from build123d import *

# Parameters (mm, degrees)
F1_DEPTH = 2


with BuildPart() as f1:
    # F0 (on Front) → F1 (new body)
    with BuildSketch(Plane.XZ):
        with BuildLine():
            Line((-13.003751, 47.985914), (-13.003751, 17.985914))
            Line((-13.003751, 17.985914), (-13.003751, -0.014086))
            Line((-13.003751, -0.014086), (-15.003751, -0.014086))
            Line((-15.003751, -0.014086), (-15.003751, 8.985914))
            Line((-15.003751, 8.985914), (-17.003751, 8.985914))
            ThreePointArc((-17.003751, 8.985914), (-18.417965, 8.400127), (-19.003751, 6.985914))
            Line((-19.003751, 6.985914), (-19.003751, -6.014086))
            Line((-19.003751, -6.014086), (-20.003751, -6.014086))
            Line((-20.003751, -6.014086), (-20.003751, -8.764086))
            Line((-20.003751, -8.764086), (-25.003751, -8.764086))
            ThreePointArc((-25.003751, -8.764086), (-26.417965, -9.349873), (-27.003751, -10.764086))
            Line((-27.003751, -10.764086), (-27.003751, -13.014086))
            Line((-27.003751, -13.014086), (-21.003751, -13.014086))
            Line((-21.003751, -13.014086), (-21.003751, -15.014086))
            Line((-21.003751, -15.014086), (-27.003751, -15.014086))
            Line((-27.003751, -15.014086), (-27.003751, -17.264086))
            ThreePointArc((-27.003751, -17.264086), (-26.417965, -18.6783), (-25.003751, -19.264086))
            Line((-25.003751, -19.264086), (-18.877196, -19.264086))
            Line((-18.877196, -19.264086), (-18.877196, -22.014086))
            Line((-18.877196, -22.014086), (-15.003751, -22.014086))
            ThreePointArc((-15.003751, -22.014086), (-13.589538, -21.4283), (-13.003751, -20.014086))
            Line((-13.003751, -20.014086), (-13.003751, -16.266214))
            ThreePointArc((-13.003751, -16.266214), (-12.094926, -14.590106), (-10.194413, -14.437287))
            ThreePointArc((-10.194413, -14.437287), (1.996249, -17.014086), (14.18691, -14.437287))
            ThreePointArc((14.18691, -14.437287), (16.087423, -14.590106), (16.996249, -16.266214))
            Line((16.996249, -16.266214), (16.996249, -20.014086))
            ThreePointArc((16.996249, -20.014086), (17.582035, -21.4283), (18.996249, -22.014086))
            Line((18.996249, -22.014086), (22.869694, -22.014086))
            Line((22.869694, -22.014086), (22.869694, -19.264086))
            Line((22.869694, -19.264086), (28.996249, -19.264086))
            ThreePointArc((28.996249, -19.264086), (30.410462, -18.6783), (30.996249, -17.264086))
            Line((30.996249, -17.264086), (30.996249, -15.014086))
            Line((30.996249, -15.014086), (24.996249, -15.014086))
            Line((24.996249, -15.014086), (24.996249, -13.014086))
            Line((24.996249, -13.014086), (30.996249, -13.014086))
            Line((30.996249, -13.014086), (30.996249, -10.764086))
            ThreePointArc((30.996249, -10.764086), (30.410462, -9.349873), (28.996249, -8.764086))
            Line((28.996249, -8.764086), (23.996249, -8.764086))
            Line((23.996249, -8.764086), (23.996249, -6.014086))
            Line((23.996249, -6.014086), (22.996249, -6.014086))
            Line((22.996249, -6.014086), (22.996249, 6.985914))
            ThreePointArc((22.996249, 6.985914), (22.410462, 8.400127), (20.996249, 8.985914))
            Line((20.996249, 8.985914), (18.996249, 8.985914))
            Line((18.996249, 8.985914), (18.996249, -0.014086))
            Line((18.996249, -0.014086), (16.996249, -0.014086))
            Line((16.996249, -0.014086), (16.996249, 17.985914))
            Line((16.996249, 17.985914), (16.996249, 47.985914))
            ThreePointArc((16.996249, 47.985914), (16.410462, 49.400127), (14.996249, 49.985914))
            Line((14.996249, 49.985914), (-11.003751, 49.985914))
            ThreePointArc((-11.003751, 49.985914), (-12.417965, 49.400127), (-13.003751, 47.985914))
        make_face()
        with BuildLine():
            Line((2.996249, -12.014086), (0.996249, -12.014086))
            Line((0.996249, -12.014086), (0.996249, -9.014086))
            ThreePointArc((0.996249, -9.014086), (1.996249, -0.126604), (2.996249, -9.014086))
            Line((2.996249, -9.014086), (2.996249, -12.014086))
        make_face(mode=Mode.SUBTRACT)
        with BuildLine():
            ThreePointArc((-8.503751, 37.985914), (-7.917965, 39.400127), (-6.503751, 39.985914))
            Line((-6.503751, 39.985914), (10.496249, 39.985914))
            ThreePointArc((10.496249, 39.985914), (11.910462, 39.400127), (12.496249, 37.985914))
            Line((12.496249, 37.985914), (12.496249, 19.985914))
            ThreePointArc((12.496249, 19.985914), (11.910462, 18.5717), (10.496249, 17.985914))
            Line((10.496249, 17.985914), (-6.503751, 17.985914))
            ThreePointArc((-6.503751, 17.985914), (-7.917965, 18.5717), (-8.503751, 19.985914))
            Line((-8.503751, 19.985914), (-8.503751, 37.985914))
        make_face(mode=Mode.SUBTRACT)
    extrude(amount=F1_DEPTH)


solid = f1.part
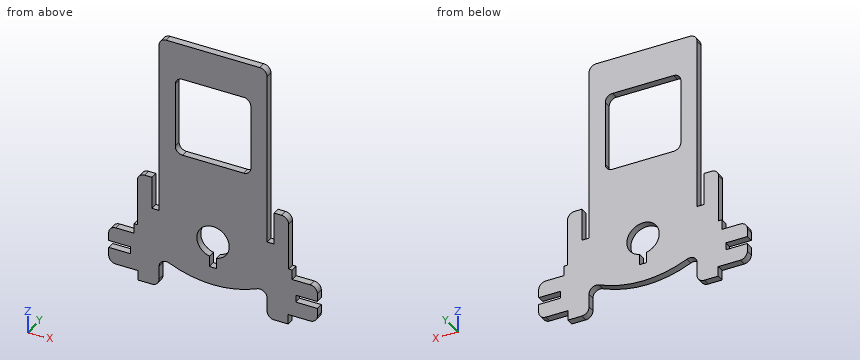
Source: CAD feature listing. Evaluate the final solid. Frame: model axes, mm. Coordinates: 2 decimals unless noted, no trailing zeros. Order: outer loops, then holes, each group sorted by start corner. A loop starts at its lowest first (then second) coordinate and runs counter-clockwise, first axis right, second up. Notation, with made-up numbers: M -7.5,-1.75 L 13.5,-1.75 A24 cw 13.5,36.25 Z; hole C 24.5,85.25 d6. An arc over 180 degrees is marked long. Write each question's results on one line, items separated by ' | '. Start each with the question number.
1. Section D-D, the plane y = -0.95. State how many separate pieces and enclosed holes the cut face has, then the cut area to 3 significant figures.
2. Section B-B, the plane z = 3. Return the cut outline in (x, y), then the cut area to 3 significant figures.
3. Pin query (flat end, axial travel): pin 1 (1 mm diameter, centred on y = -1, z = 3, fed in from -X); pin 2 (1 mm diameter, centred on y = -1.5, z = -10, fed in from +X); pin 3 (0.6 mm diameter, centred on y = -1.5, z = -20, fed in from -X). Return the tip coordinate at first contact, or that it passes through.
4. Section A-A, the plane z = 26.5. Return the cut outline in (x, y).
5. Section C-C, the plane x = 27. Return the cut outline in (y, z), then the cut area to 3 significant figures.
6. Material intervals for L1, parallel to Z at x = 2, y = -0.55; L2, parallel to X at y = -1.6, z = 38; L3, parallel to X at y = -1.65, z = 7, sorted ascending.
Solution:
1) separate pieces: 1 | enclosed holes: 2 | area: 1,920 mm²
2) outline: M -19,-2 L -15,-2 L -15,0 L -19,0 Z; M -13,-2 L 17,-2 L 17,0 L -13,0 Z; M 19,-2 L 23,-2 L 23,0 L 19,0 Z | area: 76.0 mm²
3) pin 1: x = -19 | pin 2: x = 30.98 | pin 3: x = -18.88
4) outline: M -13,-2 L -8.5,-2 L -8.5,0 L -13,0 Z; M 12.5,-2 L 17,-2 L 17,0 L 12.5,0 Z
5) outline: M -2,-19.26 L 0,-19.26 L 0,-15.01 L -2,-15.01 Z; M -2,-13.01 L 0,-13.01 L 0,-8.76 L -2,-8.76 Z | area: 17.0 mm²
6) L1: -17.01 to -12.01, -0.13 to 17.99, 39.99 to 49.99 | L2: -13 to -8.5, 12.5 to 17 | L3: -19 to -15, -13 to 17, 19 to 23
